Work out the finished part from the listing and answer in its coordinate system (mm). Face numbers are marked on the shaded views. Give positions to 0.01 mm unless a question says otherwise; leave off trailing zeros. Order: outer loops, then holes, each group sorted by start corner. A loop starts at its lowest first (then second) coordinate and runs counter-clockwise, first axis right, second up.
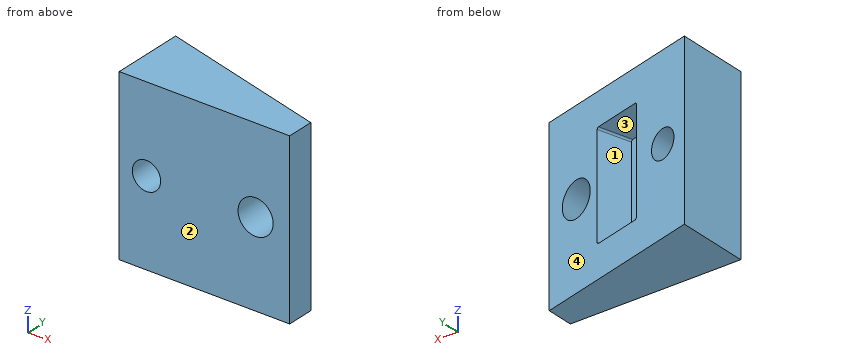
```python
from build123d import *

# Parameters (mm, degrees)
EXTRUDE_8_DEPTH     = 50
SKETCH_9_R          = 5.15
SKETCH_9_R_2        = 4.15
CUT_EXTRUDE_2_DEPTH = 50
SKETCH_10_W         = 15
SKETCH_10_H         = 31
CUT_EXTRUDE_3_DEPTH = 10
FILLET_1_R          = 0.5


with BuildPart() as part:
    # 草图8 → 凸台-拉伸8 (new body)
    with BuildSketch(Plane.XY):
        Polygon((25, -4), (25, 4), (-25, 17.397459622), (-25, 4), (-25, -4), align=None)
    extrude(amount=EXTRUDE_8_DEPTH)

    # 草图9 → 切除-拉伸2 (cut)
    with BuildSketch(Plane.XZ.offset(4)):
        with Locations(Location((15, 25, 0), (0, 0, 270))):
            Circle(SKETCH_9_R)
        with Locations(Location((-17, 25, 0), (0, 0, 270))):
            Circle(SKETCH_9_R_2)
    extrude(amount=-CUT_EXTRUDE_2_DEPTH, mode=Mode.SUBTRACT)

    # 草图10 → 切除-拉伸3 (cut)
    with BuildSketch(Plane(origin=(2.674682453, 9.982050808, 0), x_dir=(0.9659258262890701, -0.2588190451025142, 0), z_dir=(0.2588190451025142, 0.9659258262890701, 0))):
        with Locations((-2.767130523, -25)):
            Rectangle(SKETCH_10_W, SKETCH_10_H)
    extrude(amount=-CUT_EXTRUDE_3_DEPTH, mode=Mode.SUBTRACT)

    # 圆角1
    fillet_1_edges = [part.edges().sort_by_distance(p)[0] for p in [
        (-8.536699307, 7.809750594, 9.5),
        (5.952188087, 3.927464918, 9.5),
        (5.952188087, 3.927464918, 40.5),
        (-8.536699307, 7.809750594, 40.5),
    ]]
    fillet(fillet_1_edges, radius=FILLET_1_R)


solid = part.part
```
1. Given P1, Ø2, axis at x = -6, z = 21, coming from the +Y side; P2, Ø1.5, axis at x = 18.5, z = 25, coming from the +Y side; P3, Ø3, axis at x = 8.5, z = 17, coming from the +Y side, each flat-ended and moving along its own axis, determine where each tip first touches the part or whether it passes through.
Findings below:
P1: stops at y = 2.22
P2: passes through
P3: stops at y = 8.76
2. Straight lines are drawn through the part: probe 1 along Z at (x, y) = (-5.5, 11.25); probe 2 along Z at (x, y) = (-17, 1); probe 3 along X at (y, z) = (12, 23.5). For each, find the intervals that lie inside material, in ascending order.
Findings below:
probe 1: z = 0 to 9.5, 40.5 to 50
probe 2: z = 0 to 20.85, 29.15 to 50
probe 3: x = -25 to -20.87, -13.13 to -7.41
3. The part is cut by section B-B (z = 25). Write down the section's boundary in (x, y).
Findings below:
outline: (-25, -4) - (-21.15, -4) - (-21.15, 16.37) - (-25, 17.4) - close; (-12.85, -4) - (9.85, -4) - (9.85, 8.06) - (7.25, 8.76) - (4.66, -0.9) - (-9.83, 2.98) - (-7.24, 12.64) - (-12.85, 14.14) - close; (20.15, -4) - (25, -4) - (25, 4) - (20.15, 5.3) - close
4. The mould has two halves that part along X. Classify the marked faces 1, 2, 3 and 4: pulls with the +X half, pulls with the -X half, needs draft (parallel to the pull), parting line crosses it, or undercut.
Findings below:
face 1: undercut
face 2: needs draft
face 3: undercut
face 4: pulls with the +X half
5. The part is cut by section D-D (z = 32). Write down the section's boundary in (x, y), then the cut area to 3 significant figures.
Findings below:
outline: (-25, -4) - (25, -4) - (25, 4) - (7.25, 8.76) - (4.66, -0.9) - (-9.83, 2.98) - (-7.24, 12.64) - (-25, 17.4) - close
area: 585 mm2
6. The part is cut by section A-A (x = -16). Write down the section's boundary in (y, z).
Findings below:
outline: (-4, 0) - (14.99, 0) - (14.99, 20.97) - (-4, 20.97) - close; (-4, 29.03) - (14.99, 29.03) - (14.99, 50) - (-4, 50) - close
7. The part is cut by section C-C (x = 2). Write down the section's boundary in (y, z), then the cut area to 3 significant figures.
Findings below:
outline: (-4, 0) - (10.16, 0) - (10.16, 9.5) - (-0.19, 9.5) - (-0.19, 40.5) - (10.16, 40.5) - (10.16, 50) - (-4, 50) - close
area: 387 mm2
